from build123d import *

# Parameters (mm, degrees)
F1_DEPTH = 7
F3_D     = 4
F4_R     = 2


with BuildPart() as f1:
    # F0 (on Top) → F1 (new body)
    with BuildSketch(Plane.XY):
        with BuildLine():
            Line((0, 0), (0, -15))
            Line((0, -15), (6, -15))
            Line((6, -15), (6, -8))
            ThreePointArc((6, -8), (6.585786, -6.585786), (8, -6))
            Line((8, -6), (15, -6))
            Line((15, -6), (15, 0))
            Line((15, 0), (0, 0))
        make_face()
    extrude(amount=F1_DEPTH)

    # F3 (through all)
    with Locations(Plane.XY.offset(7)):
        with Locations((3, -3)):
            Hole(F3_D / 2)

    # F4
    f4_edges = [f1.edges().sort_by_distance(p)[0] for p in [
        (0, 0, 3.5),
        (0, -15, 3.5),
        (6, -15, 3.5),
        (15, -6, 3.5),
        (15, 0, 3.5),
    ]]
    fillet(f4_edges, radius=F4_R)


solid = f1.part
Model file for the job. Use its own axes, mm. A direction names the side the tool comes from. Give positions to 0.01 mm unless a question says otherwise; leave off trailing zeros. Loops run counter-clockwise (first coordinate to the right, second up) from the corner with the lowest first, then second, coordinate; pieces in that order, holes last. Notation, with made-up numbers: (66.5, -18) -> (91.5, -18) arc R13 ccw to (91.5, 1) -> close; hole circle Ø2 at (24, -25.75). An arc over 180 degrees is marked (long way). Use a Markdown table: item, result. Add a question column.
(1) Wall check: line 1 along Y through (x, z) = (3, 5.75); line 2 along Y through (x, z) = (11.5, 6); line 3 along X through (y, z) = (-1.5, 1.75). Give the ranges that are in metal, low to high.
(2) Mould opens along Y. For faces 1 (the cylindrical face through (3, -5, 3)), 2 (the flat face through (6, -6, 7)), 3 (the flat face through (3, -15, 3)) say: +Y half, -Y half, draft (parallel to the pull), parting line (faces both ways), or undercut.
(3) Slice it at B-B on x = 3. List the corners of the cut face in (y, z).
(4) Slice it at A-A on y = -3. List the corners of the cut face in (x, z), and give its area (3 significant figures).
(5) Slice it at D-D on y = -12. List the corners of the cut face in (x, z), and give its area (3 significant figures).
(6) Tool access for faces 4 (the flat face through (6, -11, 3)), 5 (the cylindrical face through (14.4, -0.57, 3.55)): list every direction of +Z, -Z, +X, -X, +Y, -Y with a clear straight run to the whole face (end or side of a thin tool).
(7) Drop flat-ended pins along their axis: pin 1 Ø4 at (x, z) = (11, 4) entering from -Y; pin 2 Ø1 at (y, z) = (-12.5, 2) entering from +X. Give the stop position or say it passes through.
(8) Slice it at C-C on z = 5.5. List the corners of the cut face in (x, y).
Filled sheet:
| question | item | result |
|---|---|---|
| 1 | line 1 | -15 to -5, -1 to 0 |
| 1 | line 2 | -6 to 0 |
| 1 | line 3 | 0.06 to 1.68, 4.32 to 14.94 |
| 2 | face 1 | undercut |
| 2 | face 2 | draft |
| 2 | face 3 | -Y half |
| 3 | outline | (-15, 0) -> (-5, 0) -> (-5, 7) -> (-15, 7) -> close; (-1, 0) -> (0, 0) -> (0, 7) -> (-1, 7) -> close |
| 4 | outline | (0, 0) -> (1, 0) -> (1, 7) -> (0, 7) -> close; (5, 0) -> (15, 0) -> (15, 7) -> (5, 7) -> close |
| 4 | area | 77.0 mm2 |
| 5 | outline | (0, 0) -> (6, 0) -> (6, 7) -> (0, 7) -> close |
| 5 | area | 42.0 mm2 |
| 6 | face 4 | +Z, -Z, +X, -Y |
| 6 | face 5 | +Z, -Z, +X, +Y |
| 7 | pin 1 | y = -6 |
| 7 | pin 2 | x = 6 |
| 8 | outline | (0, -13) arc R2 ccw to (2, -15) -> (4, -15) arc R2 ccw to (6, -13) -> (6, -8) arc R2 cw to (8, -6) -> (13, -6) arc R2 ccw to (15, -4) -> (15, -2) arc R2 ccw to (13, 0) -> (2, 0) arc R2 ccw to (0, -2) -> close; hole circle Ø4 at (3, -3) |
